from build123d import *

# Parameters (mm, degrees)
F0_R     = 33.0910363523
F1_DEPTH = 25.4
F3_D     = 25.4
F4_T     = -2.54


with BuildPart() as f1:
    # F0 (on Top) → F1 (new body)
    with BuildSketch(Plane.XY):
        with Locations((-2.0184996538, 9.1803725809)):
            Circle(F0_R)
    extrude(amount=F1_DEPTH)

    # F3 (through all)
    with Locations(Plane.XY.offset(25.4)):
        with Locations((-2.0184996538, 9.1803725809)):
            Hole(F3_D / 2)

    # F4
    f4_openings = [f1.faces().sort_by_distance(p)[0] for p in [
        (-34.17358, 9.180373, 0),
    ]]
    offset(amount=F4_T, openings=f4_openings)


solid = f1.part
The model under review builds one solid part; all positions refer to its coordinate system, in mm. A direction names the side the tool comes from. Coordinates: 2 decimals unless noted, no trailing zeros. Write each loop counter-clockwise with the first axis right and the second up, starting at its lowest first coordinate (ties: lowest second). Pieces come first, ordered by that corner, then holes. Notation, with made-up numbers: (54.5, -11) - (72.5, -11) arc R16 ccw to (72.5, 11) - close; hole circle Ø2 at (-13, 69.25). An arc over 180 degrees is marked (long way). Answer as CSV lines item,"result".
(1) We need section A-A (x = -4). Give the boundary of the cut face in (y, z), plus the area to 3 significant figures.
Data:
outline,"(-23.85, 0) - (-21.31, 0) - (-21.31, 22.86) - (-5.93, 22.86) - (-5.93, 0) - (-3.36, 0) - (-3.36, 25.4) - (-23.85, 25.4) - close; (21.72, 0) - (24.29, 0) - (24.29, 22.86) - (39.67, 22.86) - (39.67, 0) - (42.21, 0) - (42.21, 25.4) - (21.72, 25.4) - close"
area,"338 mm2"
(2) Tool access review of faces 1 (the flat face through (8, -20, 0)), 2 (the cylindrical face through (-8.641, -20.644, 11.27)): name each direction out of +Z, -Z, +X, -X, +Y, -Y from which nothing blocks a thin tool from reaching the whole face with its end or side.
Data:
face 1,"-Z, +X, -X, +Y, -Y"
face 2,"-Z"
(3) Clearance check with flat-ended pins moving along their axes: pin 1 Ø6 at (y, z) = (22, 7.5) entering from -X; pin 2 Ø12 at (y, z) = (-12, 20) entering from +X; pin 3 Ø12 at (y, z) = (7.5, 16.5) entering from +X; pin 4 Ø1.5 at (x, z) = (4, 10) entering from +Y. State where each tip first meets the part, or that it passes through.
Data:
pin 1,"stops at x = -33.62"
pin 2,"stops at x = 27.39"
pin 3,"stops at x = 31.07"
pin 4,"stops at y = 41.85"
(4) We need section B-B (y = 13). Give the boundary of the cut face in (x, z), plus the area to 3 significant figures.
Data:
outline,"(-34.89, 0) - (-32.33, 0) - (-32.33, 22.86) - (-16.77, 22.86) - (-16.77, 0) - (-14.13, 0) - (-14.13, 25.4) - (-34.89, 25.4) - close; (10.09, 0) - (12.74, 0) - (12.74, 22.86) - (28.29, 22.86) - (28.29, 0) - (30.85, 0) - (30.85, 25.4) - (10.09, 25.4) - close"
area,"343 mm2"
(5) We need section D-D (y = 36). Give the boundary of the cut face in (x, z), plus the area to 3 significant figures.
Data:
outline,"(-21.4, 0) - (-16.65, 0) - (-16.65, 22.86) - (12.61, 22.86) - (12.61, 0) - (17.37, 0) - (17.37, 25.4) - (-21.4, 25.4) - close"
area,"316 mm2"
(6) For line 1 along X through (y, z) = (-1.5, 21.5); line 2 along X through (y, z) = (13.5, 5.5); line 3 along Y through (x, z) = (-8, 15.5), list the stretches that pass through material, from the lowest coordinate up. Write a range as [from, to].
Data:
line 1,"x = [-33.34, -30.64], [-12.89, -8.89], [4.85, 8.85], [26.6, 29.3]"
line 2,"x = [-34.83, -32.26], [-16.63, -13.96], [9.92, 12.6], [28.23, 30.79]"
line 3,"y = [-23.37, -20.78], [-4.84, -2.02], [20.38, 23.2], [39.14, 41.73]"
(7) We need section C-C (z = 15). Give the boundary of the cut face in (x, y), plus the area to 3 significant figures.
Data:
outline,"circle Ø66.18 at (-2.02, 9.18); circle Ø30.48 at (-2.02, 9.18); hole circle Ø61.1 at (-2.02, 9.18); hole circle Ø25.4 at (-2.02, 9.18)"
area,"731 mm2"
(8) Mouldability with a two-part tool opening along X and no side actions: class faces 3 (the flat face through (-8, 21, 0)), 4 (the flat face through (-16, 16, 22.86)), 5 (the cylindrical face through (-35.078, 10.635, 12.522)) as pulls with the +X half, pulls with the -X half, needs draft (parallel to the pull), parting line crosses it, or undercut.
Data:
face 3,"needs draft"
face 4,"undercut"
face 5,"parting line crosses it"
